Read the model definition and answer for the solid it produces. Units are mm, in the model's axes. A direction names the side the tool comes from. Round coordinates to 2 decimals unless told otherwise and drop trailing zeros. Write each loop counter-clockwise with the first axis right and the second up, starting at its lowest first coordinate (ties: lowest second). Pieces come first, ordered by that corner, then holes. Notation, with made-up numbers: M 50.25,18.5 L 107.25,18.5 A23 ccw 107.25,35.5 Z; hole C 40.25,70 d6. An arc over 180 degrees is marked long. Use one line per item in the form item = value. Start each with the question number.
```python
from build123d import *

# Parameters (mm, degrees)
F0_W     = 76.2
F0_H     = 38.1
F1_DEPTH = 25.4
F2_SIZE  = 5.08
F3_R     = 9.525
F4_DEPTH = 12.7
F5_SIZE2 = 3.175
F5_SIZE  = 3.175
F6_T     = 7.9375


# Not quite as in the source:
# - a shell that OpenCascade refuses in one call is made with other operations: the cavity is built on its own and cut out


with BuildPart() as f1:
    # F0 (on Top) → F1 (new body)
    with BuildSketch(Plane.XY):
        with Locations((38.1, -19.05)):
            Rectangle(F0_W, F0_H)
    extrude(amount=F1_DEPTH)

    # F2
    f2_edges = [f1.edges().sort_by_distance(p)[0] for p in [
        (38.1, -38.1, 25.4),
        (76.2, -19.05, 25.4),
        (38.1, 0, 25.4),
        (0, -19.05, 25.4),
    ]]
    chamfer(f2_edges, length=F2_SIZE)

    # F3 (on face) → F4 (join)
    with BuildSketch(Plane.XY.offset(25.4)):
        with Locations((19.05, -19.05)):
            Circle(F3_R)
        with Locations((57.15, -19.05)):
            Circle(F3_R)
    extrude(amount=F4_DEPTH)

    # F5
    f5_edges = [f1.edges().sort_by_distance(p)[0] for p in [
        (9.525, -19.05, 38.1),
        (47.625, -19.05, 38.1),
    ]]
    chamfer(f5_edges, length=F5_SIZE, length2=F5_SIZE2)

    # F6: shell of thickness 7.9375, made by hand


with BuildPart() as f6_core1:
    # F6_t2: copy of F1
    add(f1.part)

    # the walls: a layer under each face that stays
    f6_faces = [f6_core1.faces().sort_by_distance(p)[0] for p in [
        (9.525, -19.05, 30.1625),
        (11.1125, -19.05, 36.5125),
        (38.1, -19.05, 25.4),
        (19.05, -19.05, 38.1),
        (38.1, -35.56, 22.86),
        (2.54, -19.05, 22.86),
        (73.66, -19.05, 22.86),
        (38.1, -2.54, 22.86),
        (47.625, -19.05, 30.1625),
        (38.1, -38.1, 10.16),
        (0, -19.05, 10.16),
        (76.2, -19.05, 10.16),
        (38.1, 0, 10.16),
        (49.2125, -19.05, 36.5125),
        (57.15, -19.05, 38.1),
    ]]
    thicken(f6_faces, amount=-F6_T, mode=Mode.SUBTRACT)

    # F6_s3 → F6_t4 (revolve, cut)
    with BuildSketch(Plane.XZ.offset(19.05)):
        Polygon((28.654375, 25.479375), (20.6375, 25.4), (20.6375, 17.4625), (28.575, 17.4625), align=None)
    revolve(axis=Axis((19.05, -19.05, 25.4), (0, 0, 1)), mode=Mode.SUBTRACT)

    # F6_s5 → F6_t6 (revolve, cut)
    with BuildSketch(Plane.XZ.offset(19.05)):
        Polygon((66.754375, 25.479375), (66.675, 17.4625), (58.7375, 17.4625), (58.7375, 25.4), align=None)
    revolve(axis=Axis((57.15, -19.05, 25.4), (0, 0, 1)), mode=Mode.SUBTRACT)


with BuildPart() as f1_1:
    add(f1.part)

    # what is left inside the walls is the cavity
    f6_cavity = [f6_core1.part.solids().sort_by_distance(p)[0] for p in [
        (38.1, -22.754167, 0.079375),
    ]]
    add(f6_cavity, mode=Mode.SUBTRACT)


solid = f1_1.part
```
Q1. Find section D-D on x = 34.5. Write down the section's boundary in (y, z), and give its area (3 significant figures).
Q2. Straight lines are drawn through the part: line 1 (X direction, y = -19, z = 27); line 2 (X direction, y = -20, z = 7); line 3 (Y direction, x = 57, z = 27). For each, find the intervals that lie inside material, in ascending order. Write a range as [from, to].
Q3. Find section B-B on x = 57.15. Write down the section's boundary in (y, z) (1 decimal).
Q4. A tool of negligible diameter and unlimited length cuts with its end or side. For faces 1 (the face through (57, -19, 30.162)), 2 (the face through (17.81, -9.606, 30.096)), 3 (the face through (38, -38.1, 10)), from which of +Z, -Z, +X, -X, +Y, -Y can it reach the whole face along a straight path? Write none if from no direction.
Q5. Find section A-A on z = 10. Write down the section's boundary in (x, y).
Q6. Each of these flat-tipped pins is pushed along its axis until it touches: pin 1 Ø6 at (x, y) = (35, -14.5) entering from -Z; pin 2 Ø2.5 at (x, y) = (57, -19) entering from -Z; pin 3 Ø17 at (x, y) = (42, -16.5) entering from -Z. Where does it stop, or does it pass through?
Q7. For a pull along X with two mould halves and no side action, classify faces 4 (the face through (76.2, -19, 10)), 5 (the face through (7.938, -19, 8)), 6 (the face through (37.57, -35.52, 22.9)) as +X half, -X half, draft (parallel to the pull), parting line (faces both ways), or undercut.
Response:
q1.outline = M -38.1,0 L -30.16,0 L -30.16,17.03 L -29.73,17.46 L -8.37,17.46 L -7.94,17.03 L -7.94,0 L 0,0 L 0,20.32 L -5.08,25.4 L -33.02,25.4 L -38.1,20.32 Z
q1.area = 554 mm²
q2.line_1 = [9.53, 17.46], [20.64, 28.57], [47.63, 55.56], [58.74, 66.67]
q2.line_2 = [0, 7.94], [68.26, 76.2]
q2.line_3 = [-28.57, -20.63], [-17.47, -9.53]
q3.outline = M -38.1,0 L -30.2,0 L -30.2,17 L -29.7,17.5 L -20.6,17.5 L -20.6,30.2 L -17.5,30.2 L -17.5,17.5 L -8.4,17.5 L -7.9,17 L -7.9,0 L 0,0 L 0,20.3 L -5.1,25.4 L -9.5,25.4 L -9.5,34.9 L -12.7,38.1 L -25.4,38.1 L -28.6,34.9 L -28.6,25.4 L -33,25.4 L -38.1,20.3 Z
q4.face_1 = -Z
q4.face_2 = +Z
q4.face_3 = +Z, -Z, +X, -X, -Y
q5.outline = M 0,-38.1 L 76.2,-38.1 L 76.2,0 L 0,0 Z; hole M 7.94,-30.16 L 68.26,-30.16 L 68.26,-7.94 L 7.94,-7.94 Z
q6.pin_1 = 17.46
q6.pin_2 = 30.16
q6.pin_3 = 17.09
q7.face_4 = +X half
q7.face_5 = undercut
q7.face_6 = draft
